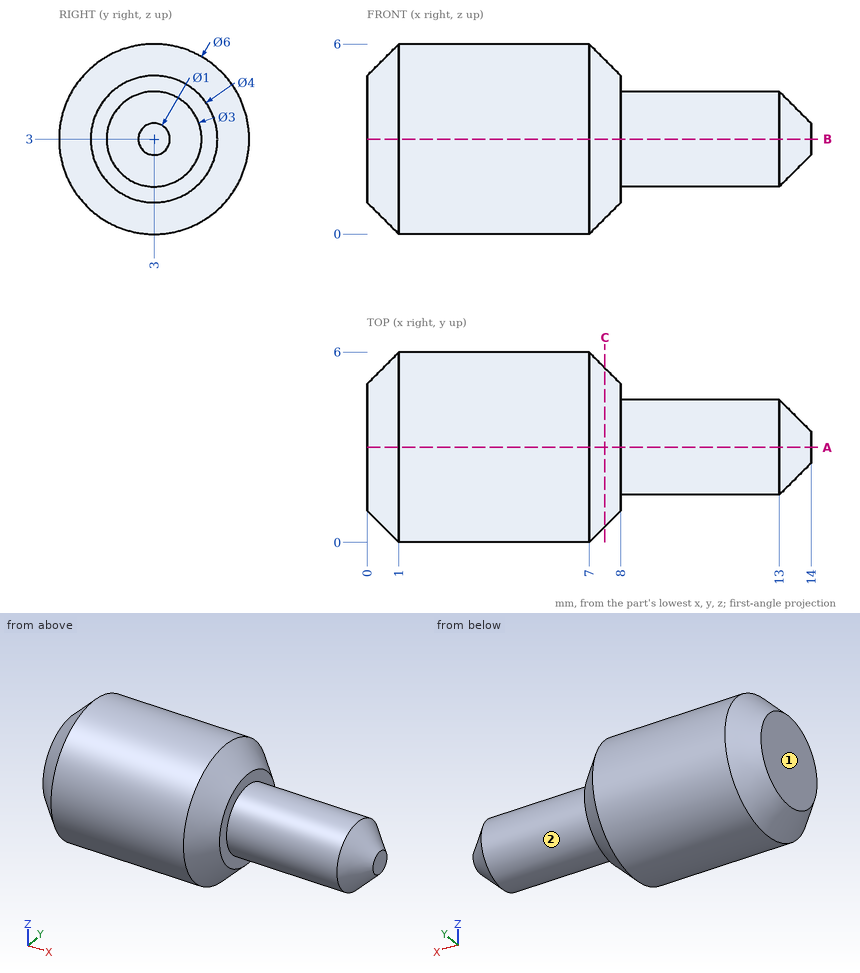
Study the drawing (mm; zero at the part's minimum x, y, z) and answer. A direction names the side the tool comes from. Coordinates: 2 decimals unless noted, no trailing zeros. Write each loop counter-clockwise with the first axis right and the second up, starting at its lowest first coordinate (ties: lowest second). Pieces come first, ordered by that corner, then holes. Notation, with made-up numbers: (-26, 77) - (16, 77) arc R31 cw to (16, 108) - close; hole circle Ø2 at (37, 56.5). An arc over 180 degrees is marked (long way). Answer as a JSON object with one key per item and string values.
Q1. Find section C-C (x = 7.5). Write down the section's boundary in (y, z).
Results list:
{"outline": "circle Ø5 at (3, 3)"}
Q2. Which of the six approach directions +Z, -Z, +X, -X, +Y, -Y give full straight-line access (tool end or side, diameter ignored) to the marked faces 1 and 2?
Results list:
{"face 1": "+Z, -Z, -X, +Y, -Y", "face 2": "+X"}
Q3. Find section A-A (y = 3). Write down the section's boundary in (x, z).
Results list:
{"outline": "(0, 1) - (1, 0) - (7, 0) - (8, 1) - (8, 1.5) - (13, 1.5) - (14, 2.5) - (14, 3.5) - (13, 4.5) - (8, 4.5) - (8, 5) - (7, 6) - (1, 6) - (0, 5) - close"}
Q4. Given pin 1 Ø1.5 at (x, z) = (7, 4.5) entering from +Y; pin 2 Ø2 at (y, z) = (4.5, 1.5) entering from +X, each flat-ended and moving along its own axis, determine where each tip first touches the part or whether it passes through.
Results list:
{"pin 1": "stops at y = 5.9", "pin 2": "stops at x = 13.38"}
Q5. Consider L1, parallel to X at y = 3.8, z = 4.8; L2, parallel to Z at x = 3, y = 5.6; L3, parallel to Z at x = 10.25, y = 2. Determine where each line is inside the solid, lowest interval first. Write a range as from..to.
Results list:
{"L1": "x = 0..8", "L2": "z = 1.5..4.5", "L3": "z = 1.88..4.12"}
